Part print with two shaded views. Sizes in mm from the minimum x, y, z corner. A direction names the side the tool comes from. Round coordinates to 2 decimals unless told otherwise and drop trailing zeros. Order: outer loops, then holes, each group sorted by start corner. A loop starts at its lowest first (then second) coordinate and runs counter-clockwise, first axis right, second up. Notation, with made-up numbers: M -37.75,21.5 L 13.25,21.5 A17 ccw 13.25,37.5 Z; hole C 77,70.25 d2. An arc over 180 degrees is marked long. Put each result on its own line as item: value.
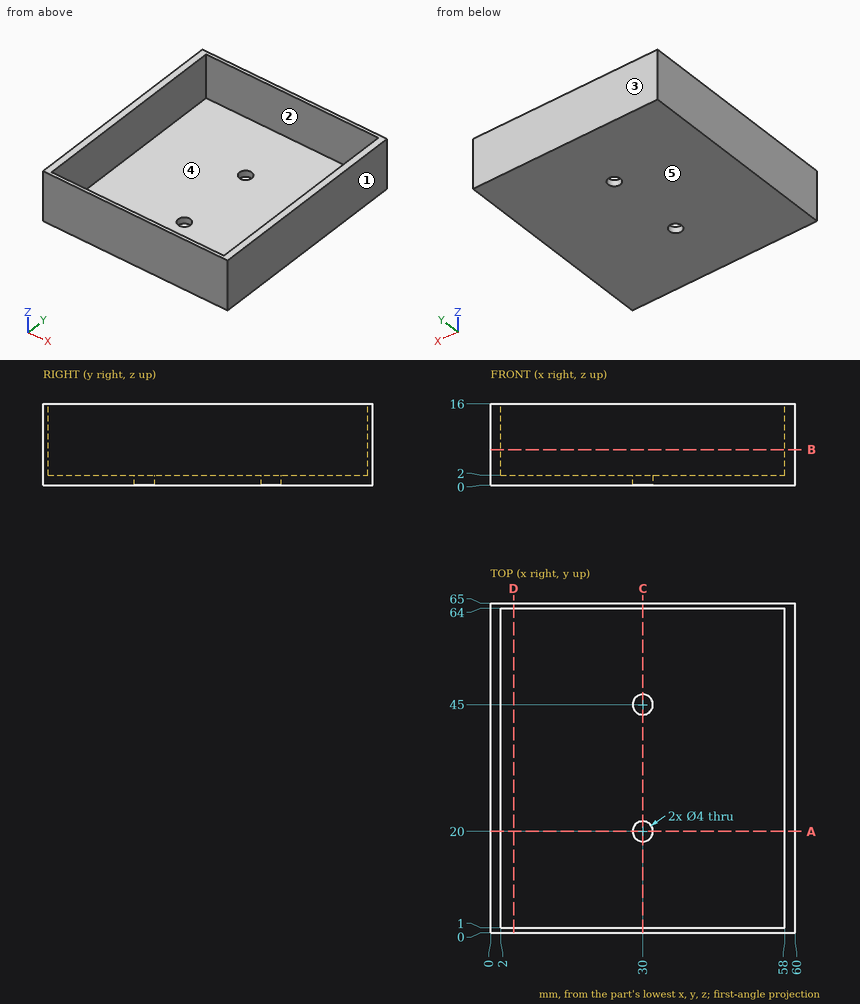
Item 1: Band-saw the part on A-A on y = 20. Give the cut face in (x, z), and give its area (3 significant figures).
Answers below:
outline: M 0,0 L 28,0 L 28,2 L 2,2 L 2,16 L 0,16 Z; M 32,0 L 60,0 L 60,16 L 58,16 L 58,2 L 32,2 Z
area: 168 mm²
Item 2: Tool access for the marked faces 4 and 5: list every direction of +Z, -Z, +X, -X, +Y, -Y with a clear straight run to the whole face (end or side of a thin tool).
Answers below:
face 4: +Z
face 5: -Z, +X, -X, +Y, -Y
Item 3: Mould opens along X. For the marked faces 1, 2 and 3 say: pulls with the +X half, pulls with the -X half, needs draft (parallel to the pull), parting line crosses it, or undercut.
Answers below:
face 1: pulls with the +X half
face 2: undercut
face 3: needs draft
Item 4: Probe line 1 along Y through (x, z) = (30, 0.9); line 2 along Y through (x, z) = (31, 12); line 3 along X through (y, z) = (39, 6.25). List the from-to ranges inside material, lowest first. Write a range as [from, to].
Answers below:
line 1: [0, 18], [22, 43], [47, 65]
line 2: [0, 1], [64, 65]
line 3: [0, 2], [58, 60]
Item 5: Band-saw the part on D-D on x = 4.5. Give the cut face in (y, z).
Answers below:
outline: M 0,0 L 65,0 L 65,16 L 64,16 L 64,2 L 1,2 L 1,16 L 0,16 Z
Item 6: Band-saw the part on C-C on x = 30. Give the cut face in (y, z), and give its area (3 significant figures).
Answers below:
outline: M 0,0 L 18,0 L 18,2 L 1,2 L 1,16 L 0,16 Z; M 22,0 L 43,0 L 43,2 L 22,2 Z; M 47,0 L 65,0 L 65,16 L 64,16 L 64,2 L 47,2 Z
area: 142 mm²
Item 7: Pin check, flat tips, straight feed: P1, Ø3, axis at x = 30, y = 20, coming from the +Z side; P2, Ø17, axis at x = 31, y = 47.5, coming from the +Z side. Stop position of each tip, or through.
Answers below:
P1: through
P2: z = 2
Item 8: Band-saw the part on B-B on z = 7. Give the cut face in (x, y).
Answers below:
outline: M 0,0 L 60,0 L 60,65 L 0,65 Z; hole M 2,1 L 58,1 L 58,64 L 2,64 Z
